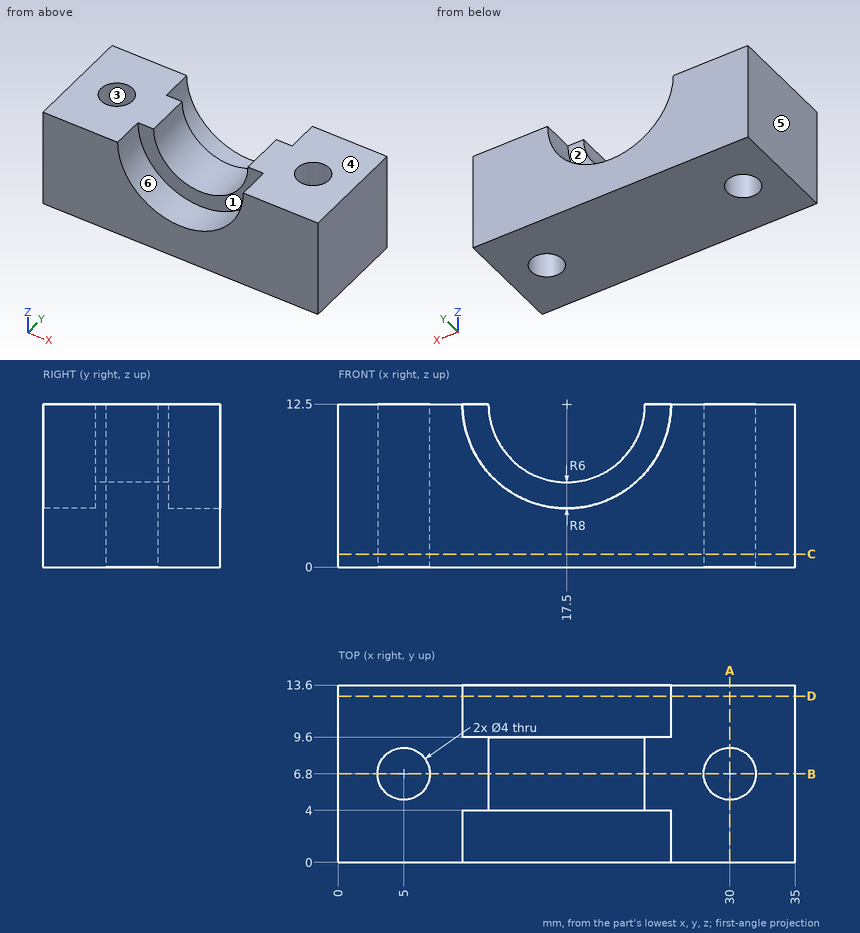
Study the drawing (mm; zero at the part's minimum x, y, z) and answer. A direction names the side the tool comes from. Round coordinates to 2 decimals unless told otherwise and drop trailing zeros. Loops run counter-clockwise (first coordinate to the right, second up) from the corner with the lowest first, then second, coordinate; pieces in that order, holes last. Notation, with made-up numbers: (76.5, -35) - (90.5, -35) arc R16 cw to (90.5, -31) - close; hole circle Ø7 at (-34, -0.5). An arc over 180 degrees is marked (long way). Use one line per item in the form item = value. Start each with the question number.
1. The part is cut by section C-C on z = 1. Determine the outline of the cut face in (x, y), then the cut area to 3 significant figures.
2. A tool of negligible diameter and unlimited length cuts with its end or side. For the marked faces 5 and 6, from which of +Z, -Z, +X, -X, +Y, -Y can it reach the whole face along a straight path? Write none if from no direction.
3. The part is cut by section A-A on x = 30. Determine the outline of the cut face in (y, z), then the cut area to 3 significant figures.
4. For a pull along Y with two mould halves and no side action, classify the marked faces 1, 2, 3 and 4 as pulls with the +Y half, pulls with the -Y half, needs draft (parallel to the pull), parting line crosses it, or undercut.
5. Consider line 1 (X direction, y = 6.8, z = 5.25); line 2 (Y direction, x = 5, z = 8.25); line 3 (X direction, y = 6.8, z = 8). Determine where each line is inside the solid, lowest interval first. Write a range as [from, to].
6. Given pin 1 Ø3 at (x, y) = (29, 8) entering from -Z; pin 2 Ø5 at (x, y) = (17.5, 3) entering from +Z; pin 3 Ø6.5 at (x, z) = (20.5, 9.5) entering from -Y, each flat-ended and moving along its own axis, determine where each tip first touches the part or whether it passes through.
7. The part is cut by section B-B on y = 6.8. Determine the outline of the cut face in (x, z), then the cut area to 3 significant figures.
8. The part is cut by section D-D on y = 12.75. Determine the outline of the cut face in (x, z), then the cut area to 3 significant figures.
Geometry check:
q1.outline = (0, 0) - (35, 0) - (35, 13.6) - (0, 13.6) - close; hole circle Ø4 at (5, 6.8); hole circle Ø4 at (30, 6.8)
q1.area = 451 mm^2
q2.face_5 = +Z, -Z, -X, +Y, -Y
q2.face_6 = +Z, -Y
q3.outline = (0, 0) - (4.8, 0) - (4.8, 12.5) - (0, 12.5) - close; (8.8, 0) - (13.6, 0) - (13.6, 12.5) - (8.8, 12.5) - close
q3.area = 120 mm^2
q4.face_1 = pulls with the -Y half
q4.face_2 = pulls with the +Y half
q4.face_3 = undercut
q4.face_4 = needs draft
q5.line_1 = [0, 3], [7, 28], [32, 35]
q5.line_2 = [0, 4.8], [8.8, 13.6]
q5.line_3 = [0, 3], [7, 13.53], [21.47, 28], [32, 35]
q6.pin_1 = 0
q6.pin_2 = 6.95
q6.pin_3 = 4
q7.outline = (0, 0) - (3, 0) - (3, 12.5) - (0, 12.5) - close; (7, 0) - (28, 0) - (28, 12.5) - (23.5, 12.5) arc R6 cw to (11.5, 12.5) - (7, 12.5) - close; (32, 0) - (35, 0) - (35, 12.5) - (32, 12.5) - close
q7.area = 281 mm^2
q8.outline = (0, 0) - (35, 0) - (35, 12.5) - (25.5, 12.5) arc R8 cw to (9.5, 12.5) - (0, 12.5) - close
q8.area = 337 mm^2
